from build123d import *

# Parameters (mm, degrees)
F0_W     = 25.4
F0_H     = 82.55
F0_H_2   = 25.4
F1_DEPTH = 25.4
F0_W_2   = 82.55
F2_DEPTH = 12.7


with BuildPart() as f1:
    # F0 (on Top) → F1 (new body)
    with BuildSketch(Plane.XY):
        with Locations((0, 53.975)):
            Rectangle(F0_W, F0_H)
        Rectangle(F0_W, F0_H_2)
        with Locations((0, -53.975)):
            Rectangle(F0_W, F0_H)
    extrude(amount=F1_DEPTH)

    # F0 (on Top) → F2 (join, symmetric)
    with BuildSketch(Plane.XY):
        with Locations((0, 53.975)):
            Rectangle(F0_W, F0_H)
        Rectangle(F0_W, F0_H_2)
        with Locations((-53.975, 0)):
            Rectangle(F0_W_2, F0_H_2)
        with Locations((53.975, 0)):
            Rectangle(F0_W_2, F0_H_2)
        with Locations((0, -53.975)):
            Rectangle(F0_W, F0_H)
    extrude(amount=F2_DEPTH, both=True)


solid = f1.part
The listing builds one solid part. Answer for the finished solid, in the listing's coordinates (mm). A direction names the side the tool comes from. Coordinates: 2 decimals unless noted, no trailing zeros. Loops run counter-clockwise (first coordinate to the right, second up) from the corner with the lowest first, then second, coordinate; pieces in that order, holes last.
1) Find section C-C on x = -69. Write down the section's boundary in (y, z), then the cut area to 3 significant figures.
2) Find section A-A on z = 10. Write down the section's boundary in (x, y).
3) Find section B-B on y = -4. Write down the section's boundary in (x, z), then the cut area to 3 significant figures.
4) A tool of negligible diameter and unlimited length cuts with its end or side. For faces 1 (the face through (53, -12.7, 0)), 2 (the face through (-55, -12.7, 0)), 3 (the face through (53, 0, 12.7)), 4 (the face through (-55, 0, 12.7)), from which of +Z, -Z, +X, -X, +Y, -Y can it reach the whole face along a straight path? Write none if from no direction.
5) Find the intervals of material crossed by L1, parallel to X at y = 44, z = 7.5, in increasing order.
6) Find section D-D on z = 20. Write down the section's boundary in (x, y).
7) Flat-ended cylindrical pins translate along their axes: pin 1 Ø8 at (y, z) = (51, 18.5) entering from -X; pin 2 Ø20.5 at (x, y) = (-44, 2.5) entering from +Z; pin 3 Ø7.5 at (x, z) = (-48, -1.5) entering from -Y. Find the tip coordinate at first contact, or state that the pin passes through.
Values:
1. outline: (-12.7, -12.7) - (12.7, -12.7) - (12.7, 12.7) - (-12.7, 12.7) - close
1. area: 645 mm2
2. outline: (-95.25, -12.7) - (-12.7, -12.7) - (-12.7, -95.25) - (12.7, -95.25) - (12.7, -12.7) - (95.25, -12.7) - (95.25, 12.7) - (12.7, 12.7) - (12.7, 95.25) - (-12.7, 95.25) - (-12.7, 12.7) - (-95.25, 12.7) - close
3. outline: (-95.25, -12.7) - (95.25, -12.7) - (95.25, 12.7) - (12.7, 12.7) - (12.7, 25.4) - (-12.7, 25.4) - (-12.7, 12.7) - (-95.25, 12.7) - close
3. area: 5,160 mm2
4. face 1: +Z, -Z, +X, -Y
4. face 2: +Z, -Z, -X, -Y
4. face 3: +Z, +X, +Y, -Y
4. face 4: +Z, -X, +Y, -Y
5. L1: x = -12.7 to 12.7
6. outline: (-12.7, -95.25) - (12.7, -95.25) - (12.7, 95.25) - (-12.7, 95.25) - close
7. pin 1: stops at x = -12.7
7. pin 2: stops at z = 12.7
7. pin 3: stops at y = -12.7
